```python
from build123d import *

# Parameters (mm, degrees)
F1_DEPTH       = 50.8
F3_D           = 6.4
F3_DEPTH       = 38.6
F3_CBORE_D     = 11.25
F3_CBORE_DEPTH = 6
F3_TIP         = 1.9227539809
F4_W           = 91.3515032281
F4_H           = 44.45
F5_DEPTH       = 180.1
F7_D           = 16
F8_R           = 6.35
F9_D           = 5
F9_CBORE_D     = 11.25
F9_CBORE_DEPTH = 6


with BuildPart() as f1:
    # F0 (on Front) → F1 (new body)
    with BuildSketch(Plane.XZ):
        with BuildLine():
            Line((-132.5, -38.8652200884), (-132.5, -82.55))
            Line((-132.5, -82.55), (132.5, -82.55))
            Line((132.5, -82.55), (132.5, -38.8652200884))
            ThreePointArc((132.5, -38.8652200884), (131.7135236391, -34.4654525376), (129.4515032281, -30.610616195))
            Line((129.4515032281, -30.610616195), (41.1484967719, 72.635616195))
            ThreePointArc((41.1484967719, 72.635616195), (38.8864763609, 76.4904525376), (38.1, 80.8902200884))
            Line((38.1, 80.8902200884), (38.1, 93.182))
            Line((38.1, 93.182), (1.5875, 93.182))
            Line((1.5875, 93.182), (1.5875, 76.2))
            Line((1.5875, 76.2), (25.4, 76.2))
            Line((25.4, 76.2), (25.4, -76.2))
            Line((25.4, -76.2), (-25.4, -76.2))
            Line((-25.4, -76.2), (-25.4, 76.2))
            Line((-25.4, 76.2), (-1.5875, 76.2))
            Line((-1.5875, 76.2), (-1.5875, 93.182))
            Line((-1.5875, 93.182), (-38.1, 93.182))
            Line((-38.1, 93.182), (-38.1, 80.8902200884))
            ThreePointArc((-38.1, 80.8902200884), (-38.8864763609, 76.4904525376), (-41.1484967719, 72.635616195))
            Line((-41.1484967719, 72.635616195), (-129.4515032281, -30.610616195))
            ThreePointArc((-129.4515032281, -30.610616195), (-131.7135236391, -34.4654525376), (-132.5, -38.8652200884))
        make_face()
    extrude(amount=F1_DEPTH)

    # F3
    with Locations(Plane(origin=(-38.1, 0, 0), x_dir=(0, -1, 0), z_dir=(-1, 0, 0))):
        with Locations((12.7, 87.0361100442), (38.1, 87.0361100442)):
            CounterBoreHole(F3_D / 2, F3_CBORE_D / 2, F3_CBORE_DEPTH, depth=F3_DEPTH)
            with Locations((0, 0, -(F3_DEPTH + F3_TIP / 2))):  # 118° drill point
                Cone(0, F3_D / 2, F3_TIP, mode=Mode.SUBTRACT)

    # F4 (on face) → F5 (cut)
    with BuildSketch(Plane.XY.offset(-76.2)):
        with Locations((86.8242483859, -25.4)):
            Rectangle(F4_W, F4_H)
        with Locations((-86.8242483859, -25.4)):
            Rectangle(F4_W, F4_H)
    extrude(amount=F5_DEPTH, mode=Mode.SUBTRACT)

    # F7 (through all)
    with Locations(Plane(origin=(0, 0, -82.55), x_dir=(1, 0, 0), z_dir=(0, 0, -1))):
        with Locations((-115, 25.4), (115, 25.4)):
            Hole(F7_D / 2)

    # F8
    f8_edges = [f1.edges().sort_by_distance(p)[0] for p in [
        (86.824248, -3.175, -76.2),
        (41.148497, -3.175, -1.782192),
        (41.148497, -25.4, -76.2),
        (86.824248, -47.625, -76.2),
        (41.148497, -47.625, -1.782192),
        (-41.148497, -25.4, -76.2),
        (-86.824248, -47.625, -76.2),
        (-41.148497, -47.625, -1.782192),
        (-86.824248, -3.175, -76.2),
        (-41.148497, -3.175, -1.782192),
    ]]
    fillet(f8_edges, radius=F8_R)

    # F9 (through all)
    with Locations(Plane(origin=(-38.1, 0, 0), x_dir=(0, -1, 0), z_dir=(-1, 0, 0))):
        with Locations((12.7, 87.0361100442), (38.1, 87.0361100442)):
            CounterBoreHole(F9_D / 2, F9_CBORE_D / 2, F9_CBORE_DEPTH)


solid = f1.part
```
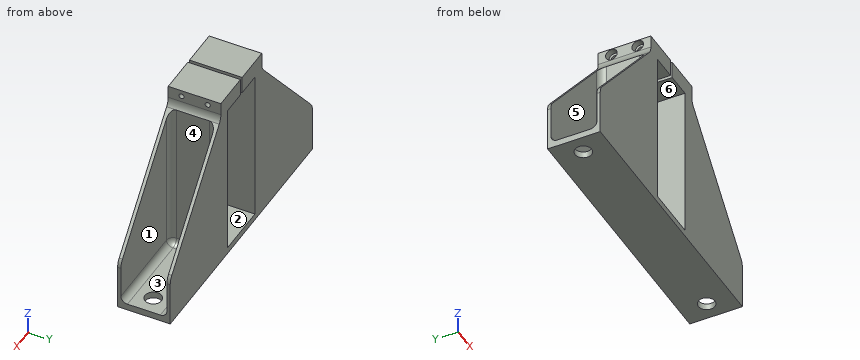
Design review of the part built by this model. Coordinates are the model's own, in mm. Face numbers are marked on the shaded views. A direction names the side the tool comes from. Round coordinates to 2 decimals unless told otherwise and drop trailing zeros. Write each loop counter-clockwise with the first axis right and the second up, starting at its lowest first coordinate (ties: lowest second). Pieces come first, ordered by that corner, then holes.
Item 1: The part is to be moulded in two halves that separate along Z. For the marked faces 1, 2 and 3, say which applies: +Z half, -Z half, draft (parallel to the pull), parting line (faces both ways), or undercut.
Item 2: We need section B-B on x = 115. Write out the cut boundary in (y, z) (3 decimals).
Item 3: For the marked faces 4, 5 and 6, list the 3-axis set-ups (+Z, -Z, +X, -X, +Y, -Y) from which the entire face can be reached by the end or side of a thin tool; tool diameter is ignored.
Item 4: For probe 1 along Z at (x, y) = (-34.45, -38.1); probe 2 along Z at (x, y) = (-21.5, -48); probe 3 along Y at (x, z) = (50, -66) (3 decimals), list the stretches that pass through material, from the lowest coordinate up.
Item 5: Clearance check with flat-ended pins moving along their axes: pin 1 Ø1 at (y, z) = (-41, 71) entering from +X; pin 2 Ø1.5 at (x, y) = (48, -5.5) entering from +Z; pin 3 Ø8.5 at (y, z) = (-38.1, 87.04) entering from +X; pin 4 Ø3.5 at (y, z) = (-37.5, 87) entering from -X. State where each tip first meets the part, or that it passes through.
Returned:
1. face 1: draft
1. face 2: undercut
1. face 3: +Z half
2. outline: (-50.8, -82.55) - (-33.4, -82.55) - (-33.4, -76.2) - (-41.275, -76.2) arc R6.35 cw to (-47.625, -69.85) - (-47.625, -13.714) - (-50.8, -13.714) - close; (-17.4, -82.55) - (0, -82.55) - (0, -13.714) - (-3.175, -13.714) - (-3.175, -69.85) arc R6.35 cw to (-9.525, -76.2) - (-17.4, -76.2) - close
3. face 4: +Z, +X
3. face 5: +Z, -X
3. face 6: +Y, -Y
4. probe 1: z = -82.55 to 81.41, 92.66 to 93.18
4. probe 2: z = -82.55 to -76.2, 76.2 to 93.18
4. probe 3: y = -50.8 to -47.625, -3.175 to 0
5. pin 1: stops at x = 41.15
5. pin 2: stops at z = -74.04
5. pin 3: stops at x = 38.1
5. pin 4: passes through
